Autodesk Fusion 360 part; units mm, degrees
sketch "Schizzo1" plane through (0, 0, 0) normal (0, 0, 1) x (1, 0, 0)
  line L0 (37.9329, 75.2335) -> (67.9329, 75.2335)
  line L1 (67.9329, 75.2335) -> (67.9329, -10.7665)
  line L2 (67.9329, -10.7665) -> (37.9329, -10.7665)
  line L3 (37.9329, -10.7665) -> (37.9329, 75.2335)
  line L4 (37.9329, -7.7665) -> (67.9329, -7.7665) construction
  line L5 (52.9329, 75.2335) -> (52.9329, -10.7665) construction
  line L6 (37.9329, 72.2335) -> (67.9329, 72.2335)
  circle A0 centre (52.9329, -7.7665) radius 1.6
  line L7 (37.9329, -4.7665) -> (67.9329, -4.7665) construction
  dimension "d1" = 30
  dimension "d3" = 3
  dimension "d4" = 3
  dimension "d5" = 3.2
  dimension "d13" = 6
  dimension "d14" = 77
extrude "Estrusione1" add sketch "Schizzo1" along normal blind 3 contours L1 L2 L3 L6 | A0
extrude "Estrusione2" add sketch "Schizzo1" along normal blind 30 contours L0 L1 L3 L6
Here's how the part is built. I have some questions about the finished solid (model axes, mm). A direction names the side the tool comes from. Give positions to 0.01 mm unless a question says otherwise; leave off trailing zeros. Loops run counter-clockwise (first coordinate to the right, second up) from the corner with the lowest first, then second, coordinate; pieces in that order, holes last. Notation, with made-up numbers: (52.25, -26.75) -> (108.25, -26.75) arc R36 ccw to (108.25, 7.25) -> close; hole circle Ø6 at (39.5, 41). An arc over 180 degrees is marked (long way). Answer as a JSON object with one key per item and string values. Group by question number.
Item 1: Imagine slicing it at B-B on z = 21. Write out the boundary of the cut face in (x, y), then the cut area to 3 significant figures.
Item 2: Imagine slicing it at C-C on y = 22.5. Write out the boundary of the cut face in (x, z), then the cut area to 3 significant figures.
Item 3: Imagine slicing it at A-A on x = 50. Write out the boundary of the cut face in (y, z), then the cut area to 3 significant figures.
Item 4: Will these pins go through, and if not, where does the flat tip stop? pin 1 (10 mm diameter, centred on x = 58.5, z = 20.5, fed in from -Y); pin 2 (2 mm diameter, centred on x = 56.5, y = 54, fed in from +Z).
Item 5: I need wall thicknesses on L1, parallel to Z at x = 57, y = 4.5; L2, parallel to Y at x = 64.5, z = 3.5. Which ranges of each line are inside material? Lowest first, please.
Item 6: On a 3-axis mill with a long thin cutter (end or side, diameter ignored), from which of +Z, -Z, +X, -X, +Y, -Y can I reach the whole of each face in a straight line? I mean faces 1 (the flat face through (53, 72.234, 16)), 2 (the flat face through (37.933, 42, 2)). Say none if no direction works.
Answer list:
{
 "1": {"outline": "(37.93, 72.23) -> (67.93, 72.23) -> (67.93, 75.23) -> (37.93, 75.23) -> close", "area": "90.0 mm2"},
 "2": {"outline": "(37.93, 0) -> (67.93, 0) -> (67.93, 3) -> (37.93, 3) -> close", "area": "90.0 mm2"},
 "3": {"outline": "(-10.77, 0) -> (75.23, 0) -> (75.23, 30) -> (72.23, 30) -> (72.23, 3) -> (-10.77, 3) -> close", "area": "339 mm2"},
 "4": {"pin 1": "stops at y = 72.23", "pin 2": "stops at z = 3"},
 "5": {"L1": "z = 0 to 3", "L2": "y = 72.23 to 75.23"},
 "6": {"face 1": "+Z, +X, -X, -Y", "face 2": "+Z, -Z, -X, +Y, -Y"}
}
